```python
from build123d import *

# Parameters (mm, degrees)
ESQUISSE1_R             = 26.25
BOSS_EXTRU_1_DEPTH      = 5
ESQUISSE2_R             = 1.5
ENL_V_MAT_EXTRU_1_DEPTH = 5
ENL_V_START             = -5
ESQUISSE3_R             = 26.25
ESQUISSE3_R_2           = 2
ENL_V_MAT_EXTRU_2_DEPTH = 5
CONG_1_R                = 2
ESQUISSE4_R             = 1.125
ENL_V_MAT_EXTRU_3_DEPTH = 10


with BuildPart() as part:
    # Esquisse1 → Boss.-Extru.1 (new body)
    with BuildSketch(Plane.XY):
        Circle(ESQUISSE1_R)
    extrude(amount=BOSS_EXTRU_1_DEPTH)

    # Esquisse2 → Enlèv. mat.-Extru.1 (cut)
    with BuildSketch(Plane.XY.offset(5)):
        Circle(ESQUISSE2_R)
    extrude(amount=-ENL_V_MAT_EXTRU_1_DEPTH, mode=Mode.SUBTRACT)

    # Esquisse3 → Enlèv. mat.-Extru.2 (cut)
    # profile 1 of 2: a face of its own
    with BuildSketch(Plane.XY.offset(5).offset(ENL_V_START)):
        Circle(ESQUISSE3_R)
        with BuildLine():
            Line((9, -2.5), (4, -2.5))
            Line((4, -2.5), (4, -19.5))
            ThreePointArc((4, -19.5), (0, -23.5), (-4, -19.5))
            Line((-4, -19.5), (-4, -2.5))
            Line((-4, -2.5), (-9, -2.5))
            ThreePointArc((-9, -2.5), (-11.5, 0), (-9, 2.5))
            Line((-9, 2.5), (-3.122498999, 2.5))
            ThreePointArc((-3.122498999, 2.5), (-2.828427125, 2.828427125), (-2.5, 3.122498999))
            Line((-2.5, 3.122498999), (-2.5, 9))
            ThreePointArc((-2.5, 9), (0, 11.5), (2.5, 9))
            Line((2.5, 9), (2.5, 3.122498999))
            ThreePointArc((2.5, 3.122498999), (2.828427125, 2.828427125), (3.122498999, 2.5))
            Line((3.122498999, 2.5), (9, 2.5))
            ThreePointArc((9, 2.5), (11.5, 0), (9, -2.5))
        make_face(mode=Mode.SUBTRACT)
    # profile 2 of 2: a face of its own
    with BuildSketch(Plane.XY.offset(5).offset(ENL_V_START)):
        with Locations((0, -19.5)):
            Circle(ESQUISSE3_R_2)
    extrude(amount=ENL_V_MAT_EXTRU_2_DEPTH, mode=Mode.SUBTRACT)

    # Congé1
    # the kernel refuses this fillet: 2 mm, written as the material it adds along each edge
    with BuildSketch(Plane(origin=(-4, -2.5, 0), x_dir=(0, -1, 0), z_dir=(0, 0, 1)), Plane(origin=(4, -2.5, 0), x_dir=(1, 0, 0), z_dir=(0, 0, 1))) as cong_1_piece_1:
        with BuildLine():
            CenterArc((CONG_1_R, -CONG_1_R), CONG_1_R, 90, 90)
            Line((0, -CONG_1_R), (0, 0))
            Line((0, 0), (CONG_1_R, 0))
        make_face()
    extrude(amount=5)
    with BuildSketch(Plane(origin=(-3.122498999, 2.5, 0), x_dir=(-1, 0, 0), z_dir=(0, 0, 1))) as cong_1_piece_2:
        with BuildLine():
            CenterArc((0.846127967, -2), CONG_1_R, 90, 41.409622109)
            ThreePointArc((-0.476747688, -0.5), (-0.227558946, -0.260311955), (0, 0))
            Line((0, 0), (0.846127967, 0))
        make_face()
    extrude(amount=5)
    with BuildSketch(Plane(origin=(-2.5, 3.122498999, 0), x_dir=(-0.7237350132500174, -0.6900779887780779, 0), z_dir=(0, 0, 1)), Plane(origin=(3.122498999, 2.5, 0), x_dir=(-0.6900779887780603, 0.7237350132500343, 0), z_dir=(0, 0, 1))) as cong_1_piece_3:
        with BuildLine():
            CenterArc((0.863575741, -1.992528413), CONG_1_R, 94.954095219, 41.409622109)
            Line((-0.583894286, -0.612372436), (0, 0))
            ThreePointArc((0, 0), (0.345430296, -0.014943173), (0.690860592, 0))
        make_face()
    extrude(amount=5)
    with BuildSketch(Plane(origin=(2.5, 3.122498999, 0), x_dir=(0.7237350132500171, -0.6900779887780782, 0), z_dir=(0, 0, 1))) as cong_1_piece_4:
        with BuildLine():
            CenterArc((0.863575741, 1.992528413), CONG_1_R, 223.636282672, 41.409622109)
            Line((-0.583894286, 0.612372436), (0, 0))
            ThreePointArc((0, 0), (0.345430296, 0.014943173), (0.690860592, 0))
        make_face()
    extrude(amount=5)

    # Esquisse4 → Enlèv. mat.-Extru.3 (cut)
    with BuildSketch(Plane.XY.offset(5)):
        with Locations((-8, 0)):
            Circle(ESQUISSE4_R)
        with Locations((8, 0)):
            Circle(ESQUISSE4_R)
        with Locations((0, 8)):
            Circle(ESQUISSE4_R)
    extrude(amount=-ENL_V_MAT_EXTRU_3_DEPTH, mode=Mode.SUBTRACT)


solid = part.part
```
Here's how the part is built. I have some questions about the finished solid (model axes, mm). A direction names the side the tool comes from. Coordinates: 2 decimals unless noted, no trailing zeros. Order: outer loops, then holes, each group sorted by start corner. A loop starts at its lowest first (then second) coordinate and runs counter-clockwise, first axis right, second up. Notation, with made-up numbers: (85, 43) -> (89, 43) arc R22 ccw to (89, 67) -> close; hole circle Ø10 at (-28.5, 74). An arc over 180 degrees is marked (long way). Return JSON: item names as keys, results as strings.
1) If we section it at A-A on y = 0: List the corners of the cut face in (x, z) for me (3 decimals).
Conclusion:
{"outline": "(-11.5, 0) -> (-9.125, 0) -> (-9.125, 5) -> (-11.5, 5) -> close; (-6.875, 0) -> (-1.5, 0) -> (-1.5, 5) -> (-6.875, 5) -> close; (1.5, 0) -> (6.875, 0) -> (6.875, 5) -> (1.5, 5) -> close; (9.125, 0) -> (11.5, 0) -> (11.5, 5) -> (9.125, 5) -> close"}
2) If we section it at C-C on x = 0: List the corners of the cut face in (y, z) for me (3 decimals).
Conclusion:
{"outline": "(-23.5, 0) -> (-21.5, 0) -> (-21.5, 5) -> (-23.5, 5) -> close; (-17.5, 0) -> (-1.5, 0) -> (-1.5, 5) -> (-17.5, 5) -> close; (1.5, 0) -> (6.875, 0) -> (6.875, 5) -> (1.5, 5) -> close; (9.125, 0) -> (11.5, 0) -> (11.5, 5) -> (9.125, 5) -> close"}
3) If we section it at D-D on z = 2.45: List the corners of the cut face in (x, y) for me (3 decimals).
Conclusion:
{"outline": "(-9, -2.5) -> (-6, -2.5) arc R2 cw to (-4, -4.5) -> (-4, -19.5) arc R4 ccw to (4, -19.5) -> (4, -4.5) arc R2 cw to (6, -2.5) -> (9, -2.5) arc R2.5 ccw to (9, 2.5) -> (3.969, 2.5) arc R2 cw to (2.845, 2.845) arc R2 cw to (2.5, 3.969) -> (2.5, 9) arc R2.5 ccw to (-2.5, 9) -> (-2.5, 3.969) arc R2 cw to (-2.845, 2.845) arc R2 cw to (-3.969, 2.5) -> (-9, 2.5) arc R2.5 ccw to start; hole circle Ø2.25 at (-8, 0); hole circle Ø4 at (0, -19.5); hole circle Ø3 at (0, 0); hole circle Ø2.25 at (0, 8); hole circle Ø2.25 at (8, 0)"}
4) If I drill on probe 1 along Y at (x, z) = (0, 2) (3 decimals); probe 2 along Y at (x, z) = (8, 3.2) (3 decimals); probe 3 along Y at (x, z) = (-6, 1.85), over which ranges is the centre line in solid material (lowest first)?
Conclusion:
{"probe 1": "y = -23.5 to -21.5, -17.5 to -1.5, 1.5 to 6.875, 9.125 to 11.5", "probe 2": "y = -2.5 to -1.125, 1.125 to 2.5", "probe 3": "y = -2.5 to 2.5"}
5) On a 3-axis mill with a long thin cutter (end or side, diameter ignored), from which of +Z, -Z, +X, -X, +Y, -Y can I reach the whole of each face in a straight line? I mean faces 1 (the flat face through (6, 2.5, 2)), 2 (the flat face through (0, -6, 0)), 3 (the flat face through (-4, -12, 2)), 4 (the flat face through (-7, 2.5, 2)). Say none if no direction works.
Conclusion:
{"face 1": "+Z, -Z, +X, +Y", "face 2": "-Z, +X, -X, +Y, -Y", "face 3": "+Z, -Z, -X, -Y", "face 4": "+Z, -Z, -X, +Y"}
6) Thinking about a two-plate mould opening in Y: for faces 5 (the cylindrical face through (0.1, -23.5, 2.5)), 6 (the cylindrical face through (-1.5, 0.07, 2.54)), 7 (the cylindrical face through (-11.5, -0.1, 2.5)), which applies, +Y half, -Y half, draft (parallel to the pull), parting line (faces both ways), or undercut?
Conclusion:
{"face 5": "-Y half", "face 6": "undercut", "face 7": "parting line"}
7) I'm going to push flat-ended pins straight in: P1, Ø3, axis at y = -2, z = 0.5, coming from the -X side; P2, Ø1.5, axis at x = -8, z = 3.5, coming from the -Y side; P3, Ø2, axis at x = -8, y = 0, coming from the -Z side; P4, Ø2.5, axis at y = -13, z = 3, coming from the +X side. Where does each tip first touch, or does it pass through?
Conclusion:
{"P1": "stops at x = -11.45", "P2": "stops at y = -2.5", "P3": "passes through", "P4": "stops at x = 4"}
8) If we section it at B-B on x = -8: List the corners of the cut face in (y, z) for me (3 decimals), plus the area to 4 significant figures.
Conclusion:
{"outline": "(-2.5, 0) -> (-1.125, 0) -> (-1.125, 5) -> (-2.5, 5) -> close; (1.125, 0) -> (2.5, 0) -> (2.5, 5) -> (1.125, 5) -> close", "area": "13.75 mm²"}
